Autodesk Inventor part; units mm, degrees
ref_plane "FDT_FRONT_XY" through (0, 0, -26.1) normal (0, 0, -1) x (1, 0, 0)
ref_plane "FDT_FRONT_YZ" through (0, 0, -26.1) normal (1, 0, 0) x (0, -1, 0)
ref_plane "FDT_FRONT_ZX" through (0, 0, -26.1) normal (0, -1, 0) x (0, 0, -1)
sketch "Sketch_12" plane through (0, 0, 0) normal (1, 0, 0) x (0, 1, 0)
  line L0 (0, -181.5) -> (0, 0)
  line L1 (0, 0) -> (14.08, 0)
  line L2 (14.08, 0) -> (15, -0.92)
  line L3 (15, -0.92) -> (15, -20.95)
  line L4 (15, -20.95) -> (14.0843, -21.8657)
  arc A0 (14.0843, -21.8657) -> (13.85, -22.4314) centre (14.65, -22.4314) ccw
  line L5 (13.85, -22.4314) -> (13.85, -23.2)
  arc A1 (13.85, -23.2) -> (14.65, -24) centre (14.65, -23.2) ccw
  line L6 (14.65, -24) -> (15, -24)
  line L7 (15, -24) -> (15, -26.1)
  line L8 (15, -26.1) -> (20.5, -26.1)
  line L9 (20.5, -26.1) -> (20.5, -45.05)
  line L10 (20.5, -45.05) -> (16.8, -45.05)
  line L11 (16.8, -45.05) -> (16.8, -136.45)
  line L12 (16.8, -136.45) -> (20.5, -136.45)
  line L13 (20.5, -136.45) -> (20.5, -155.4)
  line L14 (20.5, -155.4) -> (15, -155.4)
  line L15 (15, -155.4) -> (15, -157.5)
  line L16 (15, -157.5) -> (14.65, -157.5)
  arc A2 (14.65, -157.5) -> (13.85, -158.3) centre (14.65, -158.3) ccw
  line L17 (13.85, -158.3) -> (13.85, -159.0686)
  arc A3 (13.85, -159.0686) -> (14.0843, -159.6343) centre (14.65, -159.0686) ccw
  line L18 (14.0843, -159.6343) -> (15, -160.55)
  line L19 (15, -160.55) -> (15, -180.58)
  line L20 (15, -180.58) -> (14.08, -181.5)
  line L21 (14.08, -181.5) -> (0, -181.5)
  line L22 (0, -181.5) -> (0, 0)
revolve "Revolution1" add sketch "Sketch_12" angle 360 about axis through (0, 0, -181.5) along (0, 0, -1)
thread "Thread1"
thread "Thread2"
sketch "Sketch_1" plane through (0, 0, 0) normal (0, 0, 1) x (1, 0, 0)
  line L0 (-38, 38) -> (-38, -38)
  line L1 (-38, -38) -> (38, -38)
  line L2 (38, -38) -> (38, 38)
  line L3 (38, 38) -> (-38, 38)
  line L4 (-19, 19) -> (-19, -19)
  line L5 (-19, -19) -> (19, -19)
  line L6 (19, -19) -> (19, 19)
  line L7 (19, 19) -> (-19, 19)
extrude "Extrusion1" cut sketch "Sketch_1" against normal blind 189.5
sketch "Sketch_124" plane through (0, 0, 0) normal (0, 1, 0) x (-1, 0, 0)
  line L0 (38, -156.5) -> (8, -156.5)
  line L1 (8, -156.5) -> (8, -181.5)
  line L2 (8, -181.5) -> (-8, -181.5)
  line L3 (-8, -181.5) -> (-8, -156.5)
  line L4 (-8, -156.5) -> (-38, -156.5)
  line L5 (-38, -156.5) -> (-38, -186.5)
  line L6 (-38, -186.5) -> (38, -186.5)
  line L7 (38, -186.5) -> (38, -156.5)
extrude "Extrusion2" cut sketch "Sketch_124" along normal mid plane 38
sketch "Sketch_3" plane through (0, 0, -169.5) normal (0, 0, 1) x (1, 0, 0)
  line L0 (8, 0) -> (-8, 0)
  line L1 (-8, 0) -> (-8, 6.5774)
  line L2 (-8, 6.5774) -> (-7, 6)
  line L3 (-7, 6) -> (-6, 6)
  line L4 (-6, 6) -> (-6, 5)
  line L5 (-6, 5) -> (6, 5)
  line L6 (6, 5) -> (6, 6)
  line L7 (6, 6) -> (7, 6)
  line L8 (7, 6) -> (8, 6.5774)
  line L9 (8, 6.5774) -> (8, 0)
  line L10 (8, 0) -> (-8, 0)
revolve "Revolution2" cut sketch "Sketch_3" angle 360 about axis through (8, 0, -169.5) along (1, 0, 0)
sketch "Sketch5" plane through (-7.6974, 19, -26.1) normal (0, 1, 0) x (1, 0, 0)
  point P0 (7.6974, 9)
hole "Hole1" at (0, 19, -35.1) direction (0, -1, 0) diameter 8.566 depth 19 countersink diameter 9.728 countersink angle 90
sketch "Sketch6" plane through (-7.6974, 19, -136.45) normal (0, 1, 0) x (1, 0, 0)
  point P0 (7.6974, 9.95)
hole "Hole2" at (0, 19, -146.4) direction (0, -1, 0) diameter 8.566 depth 8.5 tip angle 120 countersink diameter 9.728 countersink angle 90
sketch "Sketch_129" plane through (0, 0, 0) normal (1, 0, 0) x (0, 1, 0)
  line L0 (0, -125) -> (0, 8)
  line L1 (0, 8) -> (6, 8)
  line L2 (6, 8) -> (6, -57)
  line L3 (6, -57) -> (16, -57)
  line L4 (16, -57) -> (16, -125)
  line L5 (16, -125) -> (0, -125)
  line L6 (0, -125) -> (0, 8)
revolve "Revolution3" cut sketch "Sketch_129" angle 360 about axis through (0, 0, -125) along (0, 0, -1)
ref_plane "FDT_FRONT_XY" through (0, 0, -26.1) normal (0, 0, -1) x (1, 0, 0)
ref_plane "FDT_FRONT_YZ" through (0, 0, -26.1) normal (1, 0, 0) x (0, -1, 0)
ref_plane "FDT_FRONT_ZX" through (0, 0, -26.1) normal (0, -1, 0) x (0, 0, -1)
ref_plane "FDT_QSFRONT_XY" through (0, 19, -35.1) normal (0, 1, 0) x (0, 0, 1)
ref_plane "FDT_QSFRONT_YZ" through (0, 19, -35.1) normal (0, 0, 1) x (1, 0, 0)
ref_plane "FDT_QSFRONT_ZX" through (0, 19, -35.1) normal (1, 0, 0) x (0, 1, 0)
ref_plane "FDT_QSREAR_XY" through (0, 19, -146.4) normal (0, 1, 0) x (0, 0, 1)
ref_plane "FDT_QSREAR_YZ" through (0, 19, -146.4) normal (0, 0, 1) x (1, 0, 0)
ref_plane "FDT_QSREAR_ZX" through (0, 19, -146.4) normal (1, 0, 0) x (0, 1, 0)
ref_plane "FDT_REAR_XY" through (0, 0, -155.4) normal (0, 0, 1) x (1, 0, 0)
ref_plane "FDT_REAR_YZ" through (0, 0, -155.4) normal (1, 0, 0) x (0, 1, 0)
ref_plane "FDT_REAR_ZX" through (0, 0, -155.4) normal (0, 1, 0) x (0, 0, 1)
ref_plane "FDT_SMBR1_XY" through (0, 0, -54.5) normal (0, 0, 1) x (-1, 0, 0)
ref_plane "FDT_SMBR1_YZ" through (0, 0, -54.5) normal (-1, 0, 0) x (0, -1, 0)
ref_plane "FDT_SMBR1_ZX" through (0, 0, -54.5) normal (0, -1, 0) x (0, 0, 1)
ref_plane "FDT_SMBR2_XY" through (0, 0, -127) normal (0, 0, 1) x (-1, 0, 0)
ref_plane "FDT_SMBR2_YZ" through (0, 0, -127) normal (-1, 0, 0) x (0, -1, 0)
ref_plane "FDT_SMBR2_ZX" through (0, 0, -127) normal (0, -1, 0) x (0, 0, 1)
ref_plane "FDT_SWIVELAXIS_XY" through (0, 0, -169.5) normal (1, 0, 0) x (0, 0, -1)
ref_plane "FDT_SWIVELAXIS_YZ" through (0, 0, -169.5) normal (0, 0, -1) x (0, 1, 0)
ref_plane "FDT_SWIVELAXIS_ZX" through (0, 0, -169.5) normal (0, 1, 0) x (1, 0, 0)
ref_plane "NUT_XY" through (0, 0, -8.5) normal (0, 0, -1) x (1, 0, 0)
ref_plane "NUT_YZ" through (0, 0, -8.5) normal (1, 0, 0) x (0, -1, 0)
ref_plane "NUT_ZX" through (0, 0, -8.5) normal (0, -1, 0) x (0, 0, -1)
ref_plane "ZR_XY" through (0, 0, 0) normal (0, 0, -1) x (-1, 0, 0)
ref_plane "ZR_YZ" through (0, 0, 0) normal (-1, 0, 0) x (0, 1, 0)
ref_plane "ZR_ZX" through (0, 0, 0) normal (0, 1, 0) x (0, 0, -1)
ref_plane "ZYL_XY" through (0, 0, -26.1) normal (0, 0, -1) x (1, 0, 0)
ref_plane "ZYL_YZ" through (0, 0, -26.1) normal (1, 0, 0) x (0, -1, 0)
ref_plane "ZYL_ZX" through (0, 0, -26.1) normal (0, -1, 0) x (0, 0, -1)
properties part number "193992 DSNU-32-60-PPS---(A----0-ZR)"
Geometry: final body of the model. Coordinates: model frame, mm. A direction names the side the tool comes from. Give positions to 0.01 mm unless a question says otherwise; leave off trailing zeros. Write each loop counter-clockwise with the first axis right and the second up, starting at its lowest first coordinate (ties: lowest second). Pieces come first, ordered by that corner, then holes.
1. Section query B-B, the plane z = -35.1. Return loops of the section in (x, y).
2. Section query A-A, the plane z = -169.5. Return loops of the section in (x, y), then the cut area to 3 significant figures.
3. Draft query along Y for faces 1 (the cylindrical face through (0.66, -14.985, -11.075)), 2 (the cylindrical face through (-15.62, -3.47, -91.48)), 3 (the flat face through (19, 0, -35)), 4 (the conical face through (-0.12, 14.24, -159.79)). Return one class per face: released by +Y, released by -Y, zero draft, split by the parting line, or undercut.
4. Pin query (flat end, axial travel): P1, Ø7.5, axis at x = 13, y = -6, coming from the -Z side; P2, Ø13, axis at y = 3, z = -168.5, coming from the -X side; P3, Ø1.5, axis at x = -12, z = -126, coming from the +Y side. Return the tip coordinate at first contact, or that it passes through.
5. Line query: probe 1 along Z at (x, y) = (0, 12); probe 2 along Z at (x, y) = (-15.5, -9.5); probe 3 along Z at (x, y) = (3, -5.5). Output: solid intervals per line, ascending.
6. Reachability of faces 5 (the cylindrical face through (0.084, 2.307, -173.936)), 6 (the flat face through (-6, -4, -166)), 7 (the flat face through (-11, -13, -45.05)) from +Z, -Z, +X, -X, +Y, -Y: full face, straight path, thin tool, end or side. Return the list, or none.
7. Section query C-C, the plane z = -74.5. Return loops of the section in (x, y), then the cut area to 3 significant figures.
Computed:
1. outline: (-19, -7.7) arc R20.5 ccw to (-7.7, -19) - (7.7, -19) arc R20.5 ccw to (19, -7.7) - (19, 7.7) arc R20.5 ccw to (7.7, 19) - (4.86, 19) - (4.28, 18.42) - (4.28, 4.2) arc R6 cw (long way) to (-4.28, 4.2) - (-4.28, 18.42) - (-4.86, 19) - (-7.7, 19) arc R20.5 ccw to (-19, 7.7) - close
2. outline: (-8, -12.69) arc R15 ccw to (8, -12.69) - (8, -6.58) - (7, -6) - (6, -6) - (6, -5) - (-6, -5) - (-6, -6) - (-7, -6) - (-8, -6.58) - close; (-8, 6.58) - (-7, 6) - (-6, 6) - (-6, 5) - (6, 5) - (6, 6) - (7, 6) - (8, 6.58) - (8, 12.69) arc R15 ccw to (-8, 12.69) - close
2. area: 287 mm2
3. face 1: split by the parting line
3. face 2: undercut
3. face 3: zero draft
3. face 4: released by +Y
4. P1: stops at z = -156.5
4. P2: stops at x = -8
4. P3: stops at y = 12.48
5. probe 1: z = -181.5 to -150.68, -142.12 to -125, -57 to -39.38, -30.82 to 0
5. probe 2: z = -155.4 to -136.45, -45.05 to -26.1
5. probe 3: z = -181.5 to -125, -57 to 0
6. face 5: +X, -X
6. face 6: -X
6. face 7: none
7. outline: circle Ø33.6 at (0, 0); hole circle Ø32 at (0, 0)
7. area: 82.4 mm2
